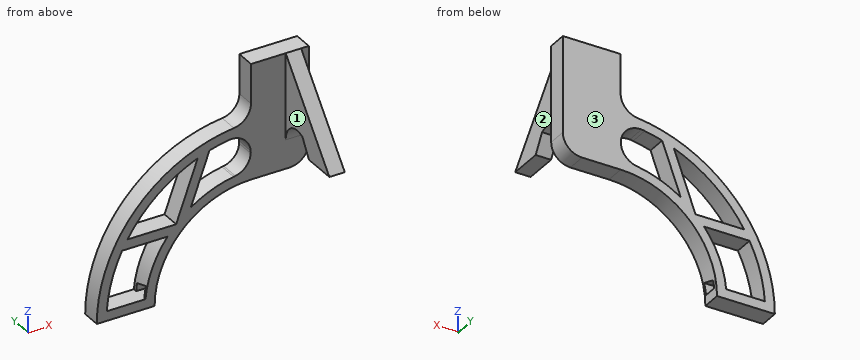
from build123d import *

# Parameters (mm, degrees)
F1_DEPTH = 10
F2_R     = 10
F4_DEPTH = 55
F6_START = -4
F6_DEPTH = 8


# Not quite as in the source:
# - a feature names something its author has since deleted; it is built from what else it names


with BuildPart() as f1:
    # F0 (on Front) → F1 (new body)
    with BuildSketch(Plane.XZ):
        with BuildLine():
            ThreePointArc((-50, 0), (-35.3553390593, 35.3553390593), (0, 50))
            Line((0, 50), (30, 50))
            Line((30, 50), (30, 110))
            Line((30, 110), (0, 110))
            Line((0, 110), (0, 89.4427191))
            ThreePointArc((0, 89.4427191), (-2.546440075, 82.7760524333), (-8.8888888889, 79.5046392))
            ThreePointArc((-8.8888888889, 79.5046392), (-59.6284794, 53.3333333333), (-80, 0))
            Line((-80, 0), (-50, 0))
        make_face()
        with BuildLine():
            Line((-0.1396715456, 63.5967118692), (-0.0513620047, 54.9999760177))
            ThreePointArc((-0.0513620047, 54.9999760177), (-4.1045972669, 54.8466250673), (-8.135508632, 54.3949767837))
            ThreePointArc((-8.135508632, 54.3949767837), (-8.5642581923, 54.317769449), (-8.9959636029, 54.2593092368))
            ThreePointArc((-8.9959636029, 54.2593092368), (-20.6018520556, 50.99572229), (-31.2178460585, 45.2818516347))
            ThreePointArc((-31.2178460585, 45.2818516347), (-35.1775050235, 42.2793464983), (-38.85, 38.9317030195))
            ThreePointArc((-38.85, 38.9317030195), (-41.1438023454, 36.4991442169), (-43.2855579864, 33.9317030195))
            ThreePointArc((-43.2855579864, 33.9317030195), (-51.1184366801, 20.2954534658), (-54.7722557505, 5))
            Line((-54.7722557505, 5), (-74.8331477355, 5))
            ThreePointArc((-74.8331477355, 5), (-72.3207331298, 19.8673490824), (-66.8852713996, 33.9317030195))
            ThreePointArc((-66.8852713996, 33.9317030195), (-65.5423309322, 36.4582344057), (-64.1039975353, 38.9317030195))
            ThreePointArc((-64.1039975353, 38.9317030195), (-48.3880483763, 57.3026768513), (-27.6441832414, 69.7194315304))
            ThreePointArc((-27.6441832414, 69.7194315304), (-24.6212334453, 70.8434532164), (-21.5527545012, 71.8364724455))
            ThreePointArc((-21.5527545012, 71.8364724455), (-17.0660687419, 73.0325221918), (-12.5139679551, 73.9486349165))
            ThreePointArc((-12.5139679551, 73.9486349165), (-11.6819966677, 74.1162256952), (-10.8388112367, 74.2126685343))
            ThreePointArc((-10.8388112367, 74.2126685343), (-5.5617429138, 74.7934958119), (-0.2568067386, 74.999560334))
            Line((-0.2568067386, 74.999560334), (-0.1540837044, 64.9997032265))
            ThreePointArc((-0.1540837044, 64.9997032265), (-0.1222411681, 64.2984606247), (-0.1396715456, 63.5967118692))
        make_face(mode=Mode.SUBTRACT)
        with BuildLine():
            ThreePointArc((-38.85, 38.9317030195), (-35.1775050235, 42.2793464983), (-31.2178460585, 45.2818516347))
            Line((-31.2178460585, 45.2818516347), (-21.5527545012, 71.8364724455))
            ThreePointArc((-21.5527545012, 71.8364724455), (-24.6212334453, 70.8434532164), (-27.6441832414, 69.7194315304))
            Line((-27.6441832414, 69.7194315304), (-38.85, 38.9317030195))
        make_face()
        with BuildLine():
            ThreePointArc((-43.2855579864, 33.9317030195), (-41.1438023454, 36.4991442169), (-38.85, 38.9317030195))
            Line((-38.85, 38.9317030195), (-64.1039975353, 38.9317030195))
            ThreePointArc((-64.1039975353, 38.9317030195), (-65.5423309322, 36.4582344057), (-66.8852713996, 33.9317030195))
            Line((-66.8852713996, 33.9317030195), (-43.2855579864, 33.9317030195))
        make_face()
        with BuildLine():
            ThreePointArc((-10.8388112367, 74.2126685343), (-3.5948385174, 71.8115750097), (-0.1540837044, 64.9997032265))
            Line((-0.1540837044, 64.9997032265), (-0.2568067386, 74.999560334))
            ThreePointArc((-0.2568067386, 74.999560334), (-5.5617429138, 74.7934958119), (-10.8388112367, 74.2126685343))
        make_face()
        with BuildLine():
            ThreePointArc((-8.135508632, 54.3949767837), (-4.1045972669, 54.8466250673), (-0.0513620047, 54.9999760177))
            Line((-0.0513620047, 54.9999760177), (-0.1396715456, 63.5967118692))
            ThreePointArc((-0.1396715456, 63.5967118692), (-2.5733550789, 57.6366041193), (-8.135508632, 54.3949767837))
        make_face()
    extrude(amount=F1_DEPTH)

    # F2
    f2_edges = [f1.edges().sort_by_distance(p)[0] for p in [
        (30, -5, 50),
    ]]
    fillet(f2_edges, radius=F2_R)

    # F3 (on Right) → F4 (cut)
    with BuildSketch(Plane.YZ):
        Polygon((-9, 11), (-9, 5), (-2, 5), (-2, 9), align=None)
    extrude(amount=-F4_DEPTH, mode=Mode.SUBTRACT)

    # F5 (on face) → F6 (join)
    with BuildSketch(Plane.YZ.offset(30).offset(F6_START)):
        with BuildLine():
            Line((-10, 65), (-10, 110))
            Line((-10, 110), (-47.6030751667, 65.1864000775))
            Line((-47.6030751667, 65.1864000775), (-30, 65))
            ThreePointArc((-30, 65), (-28.5022679561, 70.2641656131), (-24.4577120796, 73.9514693216))
            ThreePointArc((-24.4577120796, 73.9514693216), (-14.7358343869, 73.5022679561), (-10, 65))
        make_face()
        with BuildLine():
            ThreePointArc((-24.4577120796, 73.9514693216), (-28.5022679561, 70.2641656131), (-30, 65))
            add(Edge.make_bspline(
                [(-24.4577120796, 73.9514693216), (-26.3063166684, 70.9700062817), (-28.1513954112, 67.9814630399), (-30, 65)],
                knots=[0, 0, 0, 0, 10.5283312262, 10.5283312262, 10.5283312262, 10.5283312262], degree=3))
        make_face()
    extrude(amount=-F6_DEPTH)


solid = f1.part
The listing builds one solid part. Answer for the finished solid, in the listing's coordinates (mm). Face numbers are marked on the shaded views. A direction names the side the tool comes from. Coordinates: 2 decimals unless noted, no trailing zeros. Order: outer loops, then holes, each group sorted by start corner. A loop starts at its lowest first (then second) coordinate and runs counter-clockwise, first axis right, second up.
Q1. A cutting plane is placed at D-D, the plane z = 82. Write down the section's boundary in (x, y), and give its area (3 significant figures).
Q2. Which of the six approach directions +Z, -Z, +X, -X, +Y, -Y give full straight-line access (tool end or side, diameter ignored) to the marked faces 1, 2 and 3?
Q3. Consider line 1 (X direction, y = -6, z = 64) (3 decimals); line 2 (X direction, y = -42, z = 69); line 3 (Y direction, x = 14.5, z = 67.5). Determine where each line is inside the solid, lowest interval first.
Q4. A cutting plane is placed at B-B, the plane z = 28. Write down the section's boundary in (x, y).
Q5. A cutting plane is placed at C-C, the plane x = -62.5. Write down the section's boundary in (y, z), and give its area (3 significant figures).
Q6. A cutting plane is placed at A-A, the plane x = -16.5. Write down the section's boundary in (y, z).
Q7. Given P1, Ø5, axis at x = -32.5, z = 37, coming from the -Y side; P2, Ø8, axis at x = -67, y = -5, coming from the +Z side; P3, Ø8, axis at x = 14.5, y = -4, coming from the -Z side, each flat-ended and moving along its own axis, determine where each tip first touches the part or whether it passes through.
Answers follow:
1. outline: (-3.32, -10) - (18, -10) - (18, -33.49) - (26, -33.49) - (26, -10) - (30, -10) - (30, 0) - (-3.32, 0) - close
1. area: 521 mm2
2. face 1: +Z, -Z, -X, -Y
2. face 2: +Z, -Z, +X, -Y
2. face 3: +Z, -Z, +X, -X, +Y
3. line 1: x = -48 to -39.102, -29.726 to -24.405, -0.124 to 30
3. line 2: x = 18 to 26
3. line 3: y = -10 to 0
4. outline: (-74.94, -10) - (-69.58, -10) - (-69.58, 0) - (-74.94, 0) - close; (-47.34, -10) - (-41.42, -10) - (-41.42, 0) - (-47.34, 0) - close
5. outline: (-10, 0) - (0, 0) - (0, 5) - (-10, 5) - close; (-10, 33.93) - (0, 33.93) - (0, 38.93) - (-10, 38.93) - close; (-10, 41.46) - (0, 41.46) - (0, 49.94) - (-10, 49.94) - close
5. area: 185 mm2
6. outline: (-10, 47.2) - (0, 47.2) - (0, 52.47) - (-10, 52.47) - close; (-10, 73.16) - (0, 73.16) - (0, 78.28) - (-10, 78.28) - close
7. P1: stops at y = -10
7. P2: stops at z = 49.31
7. P3: stops at z = 50
